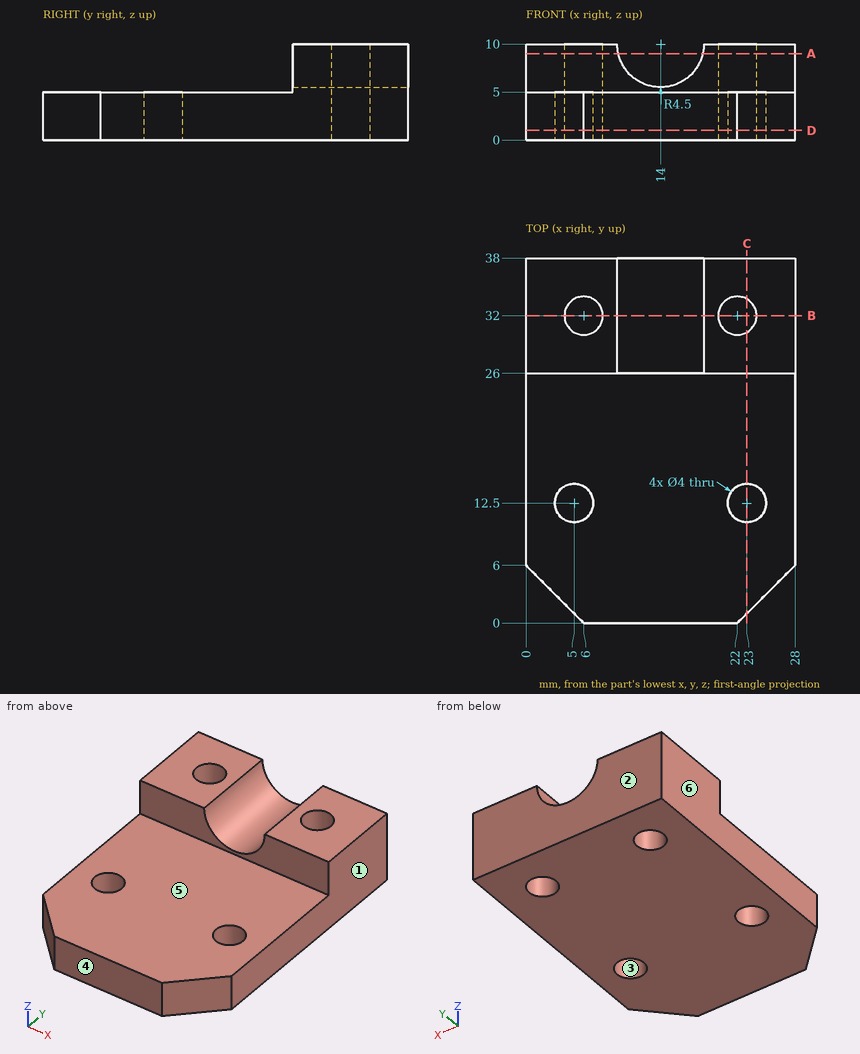
Verification items for this drawing (mm, ordinates from the low corner). A direction names the side the tool comes from. Round coordinates to 2 decimals unless told otherwise and drop trailing zeros. Order: outer loops, then holes, each group sorted by start corner. A loop starts at its lowest first (then second) coordinate and runs counter-clockwise, first axis right, second up.
1) Draft check along Y on the marked faces 1, 2, 3 and 4. Enter one of: +Y half, -Y half, draft (parallel to the pull), parting line (faces both ways), or undercut.
Geometry says:
face 1: draft
face 2: +Y half
face 3: undercut
face 4: -Y half
2) Depth check by flat-ended pin: pin 1 (4.5 mm diameter, centred on x = 5, y = 12.5, fed in from +Z); pin 2 (1.5 mm diameter, centred on x = 17.5, z = 7.5, fed in from -Y). Enter the tip coordinate at first touch or a pass-through.
Geometry says:
pin 1: stops at z = 5
pin 2: stops at y = 26
3) Cross-section at C-C, the plane x = 23. Record the cut outline in (y, z).
Geometry says:
outline: (1, 0) - (10.5, 0) - (10.5, 5) - (1, 5) - close; (14.5, 0) - (30.27, 0) - (30.27, 10) - (26, 10) - (26, 5) - (14.5, 5) - close; (33.73, 0) - (38, 0) - (38, 10) - (33.73, 10) - close
4) Cross-section at D-D, the plane z = 1. Record the cut outline in (x, y).
Geometry says:
outline: (0, 6) - (6, 0) - (22, 0) - (28, 6) - (28, 38) - (0, 38) - close; hole circle Ø4 at (5, 12.5); hole circle Ø4 at (6, 32); hole circle Ø4 at (22, 32); hole circle Ø4 at (23, 12.5)
5) Tool access check on the marked faces 5 and 6. Record the directions out of +Z, -Z, +X, -X, +Y, -Y that give a thin tool (end or side, any length) a straight path to the whole face; none if there is none.
Geometry says:
face 5: +Z, +X, -X, -Y
face 6: +Z, -Z, -X, +Y, -Y
6) Material ranges on line 1 (X direction, y = 12.5, z = 3.3); line 2 (Y direction, x = 6, z = 6.75); line 3 (Y direction, x = 6, z = 4.5), recorded low to high.
Geometry says:
line 1: x = 0 to 3, 7 to 21, 25 to 28
line 2: y = 26 to 30, 34 to 38
line 3: y = 0 to 10.77, 14.23 to 30, 34 to 38
7) Cross-section at B-B, the plane y = 32. Record the cut outline in (x, z).
Geometry says:
outline: (0, 0) - (4, 0) - (4, 10) - (0, 10) - close; (8, 0) - (20, 0) - (20, 10) - (18.5, 10) arc R4.5 cw to (9.5, 10) - (8, 10) - close; (24, 0) - (28, 0) - (28, 10) - (24, 10) - close
8) Cross-section at A-A, the plane z = 9. Record the cut outline in (x, y).
Geometry says:
outline: (0, 26) - (9.61, 26) - (9.61, 38) - (0, 38) - close; (18.39, 26) - (28, 26) - (28, 38) - (18.39, 38) - close; hole circle Ø4 at (6, 32); hole circle Ø4 at (22, 32)
